Could you check a few things on this drawing? It's one solid part, dimensions in mm from its lowest x, y, z. Coordinates: 2 decimals unless noted, no trailing zeros. Write each loop counter-clockwise with the first axis right and the second up, starting at its lowest first coordinate (ties: lowest second). Pieces come first, ordered by that corner, then holes.
Item 1: I want a section at A-A (x = 132.5). Please give me the cut outline in (y, z).
Item 2: If we mould it in two halves opening along X, with no side actions, what happens to the marked faces 1 and 2? For each: pulls with the +X half, pulls with the -X half, needs draft (parallel to the pull), parting line crosses it, or undercut.
Item 3: I want a section at B-B (z = 23). Please give me the cut outline in (x, y).
Item 4: Please list where these lines run through material, in increasing order: line 1 (Z direction, x = 7.5, y = 2.75); line 2 (X direction, y = 0.5, z = 39); line 3 (Z direction, x = 28, y = 3.5).
Item 5: I want a section at C-C (x = 112). Please give me the cut outline in (y, z), and give its area (3 significant figures).
Item 6: I'm going to push a flat-ended pin straight in: P1, Ø9, axis at x = 70, z = 25, coming from the +Y side. Where does the tip first touch, or does it pass through?
Item 7: I want a section at D-D (y = 5.5). Please give me the cut outline in (x, z), and give its area (3 significant figures).
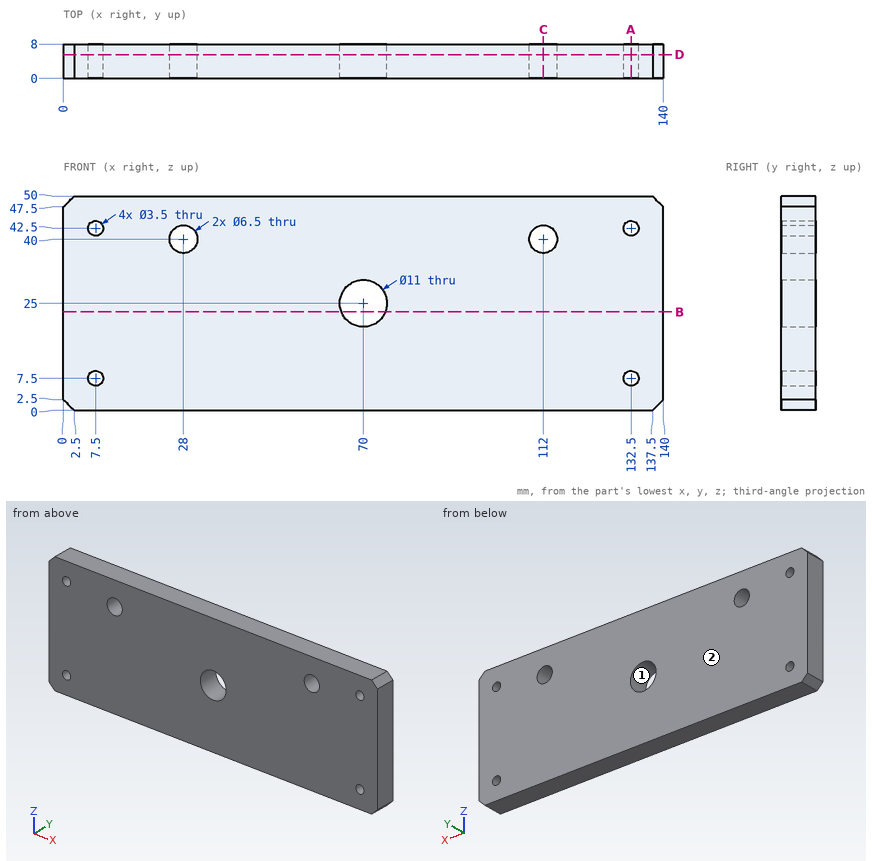
Answer:
1. outline: (0, 0) - (8, 0) - (8, 5.75) - (0, 5.75) - close; (0, 9.25) - (8, 9.25) - (8, 40.75) - (0, 40.75) - close; (0, 44.25) - (8, 44.25) - (8, 50) - (0, 50) - close
2. face 1: undercut
2. face 2: needs draft
3. outline: (0, 0) - (64.88, 0) - (64.88, 8) - (0, 8) - close; (75.12, 0) - (140, 0) - (140, 8) - (75.12, 8) - close
4. line 1: z = 0 to 5.75, 9.25 to 40.75, 44.25 to 50
4. line 2: x = 0 to 24.91, 31.09 to 108.91, 115.09 to 140
4. line 3: z = 0 to 36.75, 43.25 to 50
5. outline: (0, 0) - (8, 0) - (8, 36.75) - (0, 36.75) - close; (0, 43.25) - (8, 43.25) - (8, 50) - (0, 50) - close
5. area: 348 mm2
6. P1: passes through
7. outline: (0, 2.5) - (2.5, 0) - (137.5, 0) - (140, 2.5) - (140, 47.5) - (137.5, 50) - (2.5, 50) - (0, 47.5) - close; hole circle Ø3.5 at (7.5, 7.5); hole circle Ø3.5 at (7.5, 42.5); hole circle Ø6.5 at (28, 40); hole circle Ø11 at (70, 25); hole circle Ø6.5 at (112, 40); hole circle Ø3.5 at (132.5, 7.5); hole circle Ø3.5 at (132.5, 42.5)
7. area: 6,790 mm2
